from build123d import *

# Parameters (mm, degrees)
SKETCH_R        = 15
SKETCH_R_2      = 13.5
PAD_DEPTH       = 25
SKETCH001_W     = 5
SKETCH001_H     = 3
POCKET_DEPTH    = 10
SKETCH002_W     = 20
SKETCH002_H     = 45
PAD001_DEPTH    = 3
FILLET_R        = 4
FILLET001_R     = 4
SKETCH003_R     = 1.5
POCKET001_DEPTH = 5


with BuildPart() as part:
    # Sketch → Pad (new body)
    with BuildSketch(Plane.YZ):
        Circle(SKETCH_R)
        Circle(SKETCH_R_2, mode=Mode.SUBTRACT)
    extrude(amount=PAD_DEPTH)

    # Sketch001 (on Face4 of Pad) → Pocket (cut)
    with BuildSketch(Plane.YZ.offset(25)):
        with Locations((0, -14.5)):
            Rectangle(SKETCH001_W, SKETCH001_H)
    extrude(amount=-POCKET_DEPTH, mode=Mode.SUBTRACT)

    # Sketch002 (on DatumPlane) → Pad001 (join)
    with BuildSketch(Plane.XY.offset(17)):
        with Locations((10, 0)):
            Rectangle(SKETCH002_W, SKETCH002_H)
    extrude(amount=-PAD001_DEPTH)

    # Fillet
    fillet_edges = [part.edges().sort_by_distance(p)[0] for p in [
        (10, -5.385165, 14),
    ]]
    fillet(fillet_edges, radius=FILLET_R)

    # Fillet001
    fillet001_edges = [part.edges().sort_by_distance(p)[0] for p in [
        (10, 5.385165, 14),
    ]]
    fillet(fillet001_edges, radius=FILLET001_R)

    # Sketch003 (on Face15 of Fillet001) → Pocket001 (cut)
    with BuildSketch(Plane(origin=(0, 0, 17), x_dir=(0, -1, 0), z_dir=(0, 0, 1))):
        with Locations((-20, 10)):
            Circle(SKETCH003_R)
        with Locations((20, 10)):
            Circle(SKETCH003_R)
    extrude(amount=-POCKET001_DEPTH, mode=Mode.SUBTRACT)


solid = part.part
The model under review builds one solid part; all positions refer to its coordinate system, in mm. A direction names the side the tool comes from. Give positions to 0.01 mm unless a question says otherwise; leave off trailing zeros. Order: outer loops, then holes, each group sorted by start corner. A loop starts at its lowest first (then second) coordinate and runs counter-clockwise, first axis right, second up. Notation, with made-up numbers: M -35,23 L 10,23 A25 cw 10,43 Z; hole C 65.5,24 d1. An arc over 180 degrees is marked long. One line per question, with ' | ' between items. Start each with the question number.
1) Clearance check with flat-ended pins moving along their axes: P1, Ø1.9, axis at y = 0.5, z = -14.5, coming from the +X side; P2, Ø5, axis at x = 8.5, y = 18, coming from the -Z side; P3, Ø2, axis at x = 11.5, z = 10, coming from the -Y side. State where each tip first meets the part, or that it passes through.
2) Consider section D-D, the plane z = -11. Give the boundary of the cut face in (x, y), then the cut area to 3 significant figures.
3) Mouldability with a two-part tool opening along Z and no side actions: class faces 1 (the face through (10, 18, 14)), 2 (the face through (12.32, -2.93, -13.18)), 3 (the face through (10.07, 21.5, 15.52)), 4 (the face through (9.86, -12.69, 12)) as pulls with the +Z half, pulls with the -Z half, needs draft (parallel to the pull), parting line crosses it, or undercut.
4) For faces 5 (the face through (10, -18, 14)), 6 (the face through (20, 2.5, -14)), 7 (the face through (10, -22.5, 16)), 8 (the face through (25, -7.85, 11.21)), 9 (the face through (20, 0, 16)), list the 3-axis set-ups (+Z, -Z, +X, -X, +Y, -Y) from which the entire face can be reached by the end or side of a thin tool; tool diameter is ignored.
5) Consider section B-B, the plane x = 10. Give the boundary of the cut face in (y, z), then the cut area to 3 significant figures.
6) Consider section A-A, the plane y = 0. Give the boundary of the cut face in (x, z).
7) Consider section C-C, the plane z = 0. Give the boundary of the cut face in (x, y).
8) Wall thickness on L1, parallel to Y at x = 13.25, z = 0; L2, parallel to X at y = 20, z = 15; L3, parallel to Z at x = 21, y = 4: over which ranges is each line inside the solid? List them lowest first. Write a range as from..to.
Found:
1) P1: stops at x = 15 | P2: stops at z = 13.95 | P3: stops at y = -12.28
2) outline: M 0,-10.2 L 25,-10.2 L 25,-7.83 L 0,-7.83 Z; M 0,7.83 L 25,7.83 L 25,10.2 L 0,10.2 Z | area: 119 mm²
3) face 1: pulls with the -Z half | face 2: undercut | face 3: needs draft | face 4: undercut
4) face 5: -Z, +X, -X, -Y | face 6: -Z, +X | face 7: +Z, -Z, +X, -X, -Y | face 8: +Z, -Z, +X, +Y, -Y | face 9: +Z, +X
5) outline: M -22.5,14 L -21.5,14 L -21.5,17 L -22.5,17 Z; M -18.5,14 L -16.16,14 A4 cw -12.75,7.89 A15 ccw long 12.75,7.89 A4 cw 16.16,14 L 18.5,14 L 18.5,17 L -18.5,17 Z; M 21.5,14 L 22.5,14 L 22.5,17 L 21.5,17 Z; hole C 0,0 d27 | area: 279 mm²
6) outline: M 0,-15 L 15,-15 L 15,-13.5 L 0,-13.5 Z; M 0,13.5 L 25,13.5 L 25,15 L 20,15 L 20,17 L 0,17 Z
7) outline: M 0,-15 L 25,-15 L 25,-13.5 L 0,-13.5 Z; M 0,13.5 L 25,13.5 L 25,15 L 0,15 Z
8) L1: y = -15..-13.5, 13.5..15 | L2: x = 0..8.5, 11.5..20 | L3: z = -14.46..-12.89, 12.89..14.46
